```python
from build123d import *

# Parameters (mm, degrees)
SKETCH1_R                  = 7.9375
HEAD_DIAMETER_DEPTH        = 3.175
BOSS_EXTRUDE4_DEPTH        = 26.9748
CUT_EXTRUDE2_DEPTH         = 7.9375
SKETCH9_R                  = 4.0005
BOSS_EXTRUDE5_DEPTH        = 3.9624
SKETCH10_R                 = 2.413
CUT_EXTRUDE3_DEPTH         = 7.9248
F_10_32_TAPPED_HOLE1_D     = 4.0386
F_10_32_TAPPED_HOLE1_DEPTH = 14.224
F_10_32_TAPPED_HOLE1_TIP   = 1.213317848


with BuildPart() as part:
    # Sketch1 → Head Diameter (new body, symmetric)
    with BuildSketch(Plane(origin=(0, 0, 0), x_dir=(1, 0, 0), z_dir=(0, 1, 0))):
        Circle(SKETCH1_R)
    extrude(amount=HEAD_DIAMETER_DEPTH, both=True)

    # Sketch7 → Boss-Extrude4 (add)
    with BuildSketch(Plane(origin=(0, 0, 0), x_dir=(0, 0, -1), z_dir=(1, 0, 0))):
        with BuildLine():
            Line((-3.299361253, -3.9624), (3.299361253, -3.9624))
            ThreePointArc((3.299361253, -3.9624), (5.1562, 0), (3.299361253, 3.9624))
            Line((3.299361253, 3.9624), (-3.299361253, 3.9624))
            ThreePointArc((-3.299361253, 3.9624), (-5.1562, 0), (-3.299361253, -3.9624))
        make_face()
    extrude(amount=BOSS_EXTRUDE4_DEPTH)

    # Sketch8 → Cut-Extrude2 (cut, symmetric)
    with BuildSketch(Plane.XY):
        Polygon((0, 3.9624), (0, 3.175), (6.9342, 3.175), (7.4168, 3.9624), align=None)
        Polygon((7.4168, -3.9624), (0, -3.9624), (0, -3.175), (6.9342, -3.175), align=None)
    extrude(amount=CUT_EXTRUDE2_DEPTH, both=True, mode=Mode.SUBTRACT)

    # Sketch9 → Boss-Extrude5 (add, symmetric)
    with BuildSketch(Plane(origin=(0, 0, 0), x_dir=(1, 0, 0), z_dir=(0, 1, 0))):
        Circle(SKETCH9_R)
    extrude(amount=BOSS_EXTRUDE5_DEPTH, both=True)

    # Sketch10 → Cut-Extrude3 (cut)
    with BuildSketch(Plane(origin=(0, 3.9624, 0), x_dir=(1, 0, 0), z_dir=(0, 1, 0))):
        Circle(SKETCH10_R)
    extrude(amount=-CUT_EXTRUDE3_DEPTH, mode=Mode.SUBTRACT)

    # #10-32 Tapped Hole1
    with Locations(Plane(origin=(26.9748, 0, 0), x_dir=(0, 0, -1), z_dir=(1, 0, 0))):
        with Locations((0, 0)):
            Hole(F_10_32_TAPPED_HOLE1_D / 2, depth=F_10_32_TAPPED_HOLE1_DEPTH)
            with Locations((0, 0, -(F_10_32_TAPPED_HOLE1_DEPTH + F_10_32_TAPPED_HOLE1_TIP / 2))):  # 118° drill point
                Cone(0, F_10_32_TAPPED_HOLE1_D / 2, F_10_32_TAPPED_HOLE1_TIP, mode=Mode.SUBTRACT)


solid = part.part
```
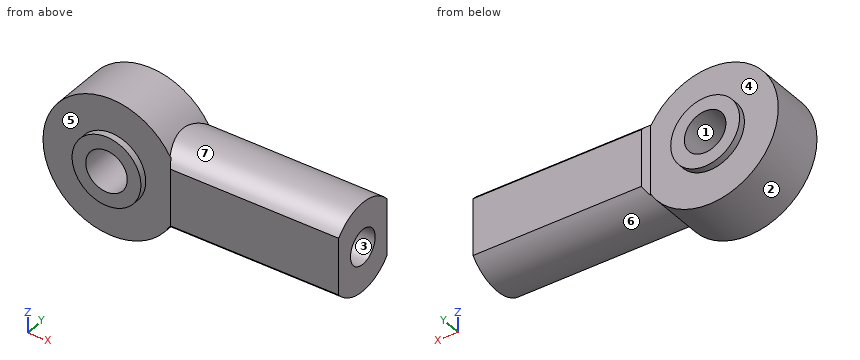
Could you check a few things on this model? Use its own coordinates, in mm. Face numbers are marked on the shaded views. A direction names the side the tool comes from. Coordinates: 2 decimals unless noted, no trailing zeros. Order: outer loops, then holes, each group sorted by start corner. A loop starts at its lowest first (then second) coordinate and runs counter-clockwise, first axis right, second up. Notation, with made-up numbers: M -6.5,24 L 46.5,24 A29 ccw 46.5,55 Z; hole C -18,13.5 d7. An arc over 180 degrees is marked long. Use one line per item in the form item = value. Start each with the question number.
1. On a 3-axis mill with a long thin cutter (end or side, diameter ignored), from which of +Z, -Z, +X, -X, +Y, -Y can I reach the whole of each face in a straight line? I mean the marked faces 4, 5, 6 and 7. Say none if no direction works.
2. We'd pull the mould along X, two halves only. Please class the marked faces 1, 2 and 3: +X half, -X half, draft (parallel to the pull), parting line (faces both ways), or undercut.
3. Suppose I cut it at C-C on x = 11. Write out the boundary of the cut face in (y, z), then the cut area to 4 significant figures.
4. For pin 1 (3 mm diameter, centred on y = 0, z = 0, fed in from +X); pin 2 (1 mm diameter, centred on x = 16.5, z = -5, fed in from -Y), each with a flat end and sliding along its axis, tell me the tip position at first contact or that it passes through.
5. Suppose I cut it at A-A on x = 0. Write out the boundary of the cut face in (y, z) (1 decimal), then the cut area to 3 significant figures.
6. Suppose I cut it at B-B on z = 4.5. Write out the boundary of the cut face in (x, y) (3 decimals).
7. Please list where these lines run through material, in increasing order: line 1 (Y direction, x = 21, z = 0); line 2 (Z direction, x = 0, y = -0.25); line 3 (Z direction, x = 20.75, y = 0).
Geometry says:
q1.face_4 = +Y
q1.face_5 = -Y
q1.face_6 = -Z, +X
q1.face_7 = +Z, +X
q2.face_1 = undercut
q2.face_2 = parting line
q2.face_3 = draft
q3.outline = M -3.96,-3.3 A5.16 ccw 3.96,-3.3 L 3.96,3.3 A5.16 ccw -3.96,3.3 Z
q3.area = 72.75 mm^2
q4.pin_1 = 12.44
q4.pin_2 = -2.52
q5.outline = M -4,-4 L -3.2,-4 L -3.2,-7.9 L 3.2,-7.9 L 3.2,-4 L 4,-4 L 4,-2.4 L -4,-2.4 Z; M -4,2.4 L 4,2.4 L 4,4 L 3.2,4 L 3.2,7.9 L -3.2,7.9 L -3.2,4 L -4,4 Z
q5.area = 75.2 mm^2
q6.outline = M -6.539,-3.175 L 6.539,-3.175 L 6.539,-2.517 L 26.975,-2.517 L 26.975,2.517 L 6.539,2.517 L 6.539,3.175 L -6.539,3.175 Z
q7.line_1 = -3.96 to -2.02, 2.02 to 3.96
q7.line_2 = -7.94 to -2.41, 2.41 to 7.94
q7.line_3 = -5.16 to -2.02, 2.02 to 5.16
